Part model, mm, in its own coordinate system. A direction names the side the tool comes from. Round coordinates to 2 decimals unless told otherwise and drop trailing zeros. Order: outer loops, then holes, each group sorted by start corner. A loop starts at its lowest first (then second) coordinate and runs counter-clockwise, first axis right, second up. Notation, with made-up numbers: (75, 28.25) - (82, 28.25) arc R20 cw to (82, 35.25) - close; hole circle Ø8 at (-26.5, 42). An arc over 180 degrees is marked (long way). Answer as a JSON object with one key per item and string values.
```python
from build123d import *

# Parameters (mm, degrees)
SHELL1_T                = -10
SKETCH4_W               = 41
SKETCH4_H               = 21
CUT_EXTRUDE1_DEPTH      = 10
SKETCH5_W               = 7.5
SKETCH5_H               = 21
CUT_EXTRUDE2_DEPTH      = 5
SKETCH6_R               = 2.16
CUT_EXTRUDE3_DEPTH      = 5
MIRROR1_COPY_1_SKETCH_R = 2.16
MIRROR1_COPY_1_DEPTH    = 5
SKETCH7_W               = 4
SKETCH7_H               = 3.5
CUT_EXTRUDE4_DEPTH      = 10
CUT_EXTRUDE7_DEPTH      = 30


with BuildPart() as part:
    # Sketch2 → Revolve1 (revolve)
    with BuildSketch(Plane.XY, mode=Mode.PRIVATE) as revolve1_sk:
        Polygon((0, 0), (0, 40), (-50, 40), (-65.896319649, 0), align=None)
    revolve(revolve1_sk.sketch.rotate(Axis((0, 0, 0), (0, 1, 0)), 270), axis=Axis((0, 0, 0), (0, 1, 0)))

    # Shell1
    shell1_openings = [part.faces().sort_by_distance(p)[0] for p in [
        (0, 0, 0),
    ]]
    offset(amount=SHELL1_T, openings=shell1_openings, kind=Kind.INTERSECTION)

    # Sketch4 → Cut-Extrude1 (cut)
    with BuildSketch(Plane(origin=(0, 40, 0), x_dir=(1, 0, 0), z_dir=(0, 1, 0))):
        Rectangle(SKETCH4_W, SKETCH4_H)
    extrude(amount=-CUT_EXTRUDE1_DEPTH, mode=Mode.SUBTRACT)

    # Sketch5 → Cut-Extrude2 (cut)
    with BuildSketch(Plane(origin=(0, 40, 0), x_dir=(1, 0, 0), z_dir=(0, 1, 0))):
        with Locations((-24.25, 0)):
            Rectangle(SKETCH5_W, SKETCH5_H)
    cut_extrude2 = extrude(amount=-CUT_EXTRUDE2_DEPTH, mode=Mode.SUBTRACT)

    # Sketch6 → Cut-Extrude3 (cut)
    with BuildSketch(Plane(origin=(0, 35, 0), x_dir=(1, 0, 0), z_dir=(0, 1, 0))):
        with Locations(Location((-24.19, 6.31, 0), (0, 0, 270))):
            Circle(SKETCH6_R)
    cut_extrude3 = extrude(amount=-CUT_EXTRUDE3_DEPTH, mode=Mode.SUBTRACT)

    # Mirror2: Cut-Extrude3 across plane
    add(cut_extrude3.mirror(Plane.XY), mode=Mode.SUBTRACT)

    # Mirror1: Cut-Extrude2, Cut-Extrude3 across plane
    add(cut_extrude2.mirror(Plane(origin=(0, 0, 0), x_dir=(0, 0, 1), z_dir=(1, 0, 0))), mode=Mode.SUBTRACT)
    add(cut_extrude3.mirror(Plane(origin=(0, 0, 0), x_dir=(0, 0, 1), z_dir=(1, 0, 0))), mode=Mode.SUBTRACT)

    # Mirror1 copy 1 sketch → Mirror1 copy 1 (cut)
    with BuildSketch(Plane(origin=(0, 35, 0), x_dir=(-1, 0, 0), z_dir=(0, 1, 0))):
        with Locations(Location((-24.19, 6.31, 0), (0, 0, 270))):
            Circle(MIRROR1_COPY_1_SKETCH_R)
    extrude(amount=-MIRROR1_COPY_1_DEPTH, mode=Mode.SUBTRACT)

    # Sketch7 → Cut-Extrude4 (cut)
    with BuildSketch(Plane(origin=(0, 35, 0), x_dir=(1, 0, 0), z_dir=(0, 1, 0))):
        with Locations((22.5, -1.75)):
            Rectangle(SKETCH7_W, SKETCH7_H)
    cut_extrude4 = extrude(amount=-CUT_EXTRUDE4_DEPTH, mode=Mode.SUBTRACT)

    # Mirror3: Cut-Extrude4 across plane
    add(cut_extrude4.mirror(Plane.XY), mode=Mode.SUBTRACT)

    # Sketch8 → Cut-Extrude7 (cut)
    with BuildSketch(Plane.XZ):
        with BuildLine():
            Line((-20, 51.38028066), (-20, 20))
            Line((-20, 20), (20, 20))
            Line((20, 20), (20, 51.38028066))
            ThreePointArc((20, 51.38028066), (0, 55.135589602), (-20, 51.38028066))
        make_face()
        with BuildLine():
            Line((-20, -51.38028066), (-20, -62.787936288))
            ThreePointArc((-20, -62.787936288), (0, -65.896319649), (20, -62.787936288))
            Line((20, -62.787936288), (20, -51.38028066))
            ThreePointArc((20, -51.38028066), (0, -55.135589602), (-20, -51.38028066))
        make_face()
        with BuildLine():
            ThreePointArc((20, 62.787936288), (0, 65.896319649), (-20, 62.787936288))
            Line((-20, 62.787936288), (-20, 51.38028066))
            ThreePointArc((-20, 51.38028066), (0, 55.135589602), (20, 51.38028066))
            Line((20, 51.38028066), (20, 62.787936288))
        make_face()
        with BuildLine():
            Line((-51.38028066, -20), (-20, -20))
            Line((-20, -20), (-20, 20))
            Line((-20, 20), (-51.38028066, 20))
            ThreePointArc((-51.38028066, 20), (-55.135589602, 0), (-51.38028066, -20))
        make_face()
        with BuildLine():
            ThreePointArc((-62.787936288, 20), (-65.896319649, 0), (-62.787936288, -20))
            Line((-62.787936288, -20), (-51.38028066, -20))
            ThreePointArc((-51.38028066, -20), (-55.135589602, 0), (-51.38028066, 20))
            Line((-51.38028066, 20), (-62.787936288, 20))
        make_face()
        with BuildLine():
            Line((51.38028066, -20), (62.787936288, -20))
            ThreePointArc((62.787936288, -20), (65.114586933, -10.12005493), (65.896319649, 0))
            ThreePointArc((65.896319649, 0), (65.114586933, 10.12005493), (62.787936288, 20))
            Line((62.787936288, 20), (51.38028066, 20))
            ThreePointArc((51.38028066, 20), (54.188630306, 10.174752396), (55.135589602, 0))
            ThreePointArc((55.135589602, 0), (54.188630306, -10.174752396), (51.38028066, -20))
        make_face()
        with BuildLine():
            Line((-20, -20), (-20, -51.38028066))
            ThreePointArc((-20, -51.38028066), (0, -55.135589602), (20, -51.38028066))
            Line((20, -51.38028066), (20, -20))
            Line((20, -20), (-20, -20))
        make_face()
        with BuildLine():
            Line((20, 20), (20, -20))
            Line((20, -20), (51.38028066, -20))
            ThreePointArc((51.38028066, -20), (54.188630306, -10.174752396), (55.135589602, 0))
            ThreePointArc((55.135589602, 0), (54.188630306, 10.174752396), (51.38028066, 20))
            Line((51.38028066, 20), (20, 20))
        make_face()
    extrude(amount=-CUT_EXTRUDE7_DEPTH, mode=Mode.SUBTRACT)


solid = part.part
```
Item 1: Cut at C-C (z = 6.31). State how many separate pieces and enclosed holes the cut face has, plus the area to 3 significant figures.
Taken from the geometry:
{"separate pieces": "4", "enclosed holes": "0", "area": "504 mm2"}
Item 2: Cut at A-A (x = 0). Write the cut outline in (y, z), plus the area to 3 significant figures.
Taken from the geometry:
{"outline": "(30, -53.97) - (40, -50) - (40, -10.5) - (30, -10.5) - close; (30, 10.5) - (40, 10.5) - (40, 50) - (30, 53.97) - close", "area": "830 mm2"}
Item 3: Drop flat-ended pins along their axis: P1, Ø7.5, axis at x = -49, y = 19.5, coming from the -Z side; P2, Ø12, axis at y = 13, z = 48, coming from the +X side; P3, Ø7.5, axis at x = -53.5, y = 8.5, coming from the +Z side. Give the stop position or say it passes through.
Taken from the geometry:
{"P1": "z = -37.09", "P2": "x = 44.75", "P3": "z = 38.44"}
Item 4: Cut at D-D (y = 10). Write the cut outline in (x, z), plus the area to 3 significant figures.
Taken from the geometry:
{"outline": "(-58.6, -20) arc R61.92 ccw to (-20, -58.6) - (-20, -47.09) arc R51.16 cw to (-47.09, -20) - close; (-58.6, 20) - (-47.09, 20) arc R51.16 cw to (-20, 47.09) - (-20, 58.6) arc R61.92 ccw to start; (20, -58.6) arc R61.92 ccw to (58.6, -20) - (47.09, -20) arc R51.16 cw to (20, -47.09) - close; (20, 47.09) arc R51.16 cw to (47.09, 20) - (58.6, 20) arc R61.92 ccw to (20, 58.6) - close", "area": "2,060 mm2"}
Item 5: Probe L1, parallel to Z at x = 24, y = 33; L2, parallel to X at y = 31.25, z = 6.31; L3, parallel to X at y = 33, z = -6. List the from-to ranges inside material, lowest first. Write a range as from..to.
Taken from the geometry:
{"L1": "-47.01..-8.46, -4.16..-3.5, 3.5..4.16, 8.46..47.01", "L2": "-53.1..-26.35, -22.03..-20.5, 20.5..22.03, 26.35..53.1", "L3": "-52.44..-26.33, -22.05..-20.5, 20.5..22.05, 26.33..52.44"}
Item 6: Two-plate mould, pull along X, no slides. Class faces 1 (the flat face through (41, 0, -41)), 2 (the flat face through (22, 33, -3.5)): pulls with the +X half, pulls with the -X half, needs draft (parallel to the pull), parting line crosses it, or undercut.
Taken from the geometry:
{"face 1": "needs draft", "face 2": "undercut"}
Item 7: Cut at B-B (y = 18). Write the cut outline in (x, z).
Taken from the geometry:
{"outline": "(-55.23, -20) arc R58.74 ccw to (-20, -55.23) - (-20, -43.62) arc R47.98 cw to (-43.62, -20) - close; (-55.23, 20) - (-43.62, 20) arc R47.98 cw to (-20, 43.62) - (-20, 55.23) arc R58.74 ccw to start; (20, -55.23) arc R58.74 ccw to (55.23, -20) - (43.62, -20) arc R47.98 cw to (20, -43.62) - close; (20, 43.62) arc R47.98 cw to (43.62, 20) - (55.23, 20) arc R58.74 ccw to (20, 55.23) - close"}
Item 8: Tool access for faces 3 (the flat face through (25, 35, 0)), 4 (the flat face through (24.5, 33, 0)), 5 (the conical face through (-35.03, 14.79, 34.63)), 6 (the flat face through (-20, 15, 51)): list every direction of +Z, -Z, +X, -X, +Y, -Y with a clear straight run to the whole face (end or side of a thin tool).
Taken from the geometry:
{"face 3": "+Y", "face 4": "+Y, -Y", "face 5": "-Y", "face 6": "+Z, -Z, -Y"}
